Autodesk Inventor part; units mm, degrees
ref_plane "YZ Plane" through (0, 0, 0) normal (1, 0, 0) x (0, 1, 0)
ref_plane "XZ Plane" through (0, 0, 0) normal (0, 1, 0) x (-1, 0, 0)
ref_plane "XY Plane" through (0, 0, 0) normal (0, 0, 1) x (1, 0, 0)
sketch "Sketch1" plane through (0, 0, 0) normal (0, 0, 1) x (1, 0, 0)
  line L0 (-21.5, 19) -> (21.5, 19)
  line L1 (21.5, 19) -> (21.5, -19)
  line L2 (21.5, -19) -> (-21.5, -19)
  line L3 (-21.5, -19) -> (-21.5, 19)
  line L4 (0, 0) -> (0, 19) construction
  line L5 (0, 0) -> (0, -19) construction
  line L6 (0, 0) -> (21.5, 0) construction
  line L7 (0, 0) -> (-21.5, 0) construction
  dimension "d0" = 43
  dimension "d1" = 38
extrude "Extrusion1" add sketch "Sketch1" along normal blind 4.5
sketch "Sketch2" plane through (0, 0, 4.5) normal (0, 0, 1) x (1, 0, 0)
  line L0 (21.5, 19) -> (21.5, -19)
  line L1 (-21.5, 19) -> (21.5, 19)
  line L2 (-21.5, -19) -> (-21.5, 19)
  line L3 (21.5, -19) -> (-21.5, -19)
  line L4 (19.7, 17.2) -> (19.7, -17.2)
  line L5 (19.7, -17.2) -> (-19.7, -17.2)
  line L6 (-19.7, -17.2) -> (-19.7, 17.2)
  line L7 (-19.7, 17.2) -> (19.7, 17.2)
  dimension "d4" = 1.8
extrude "Extrusion2" cut sketch "Sketch2" against normal blind 2.25 contours L4 L5 L6 L7
sketch "Sketch3" plane through (0, 0, 0) normal (0, 0, -1) x (-1, 0, 0)
  line L0 (21.5, 19) -> (-21.5, 19)
  line L1 (-21.5, 19) -> (-21.5, -19)
  line L2 (-21.5, 17) -> (-23.5, 17)
  line L3 (-23.5, 17) -> (-23.5, 12.725)
  line L4 (-23.5, 12.725) -> (-34.5, 12.725)
  line L5 (-34.5, 12.725) -> (-34.5, 2.425)
  line L6 (-34.5, 2.425) -> (-23.5, 2.425)
  line L7 (-23.5, 2.425) -> (-23.5, -1.85)
  line L8 (-23.5, -1.85) -> (-21.5, -1.85)
  dimension "d7" = 2
  dimension "d8" = 2
  dimension "d9" = 18.85
  dimension "d10" = 10.3
  dimension "d11" = 13
extrude "Extrusion3" add sketch "Sketch3" against normal blind 2
fillet "Fillet1" radius 5.15 2 edges at (34.5, 2.425, 1) (34.5, 12.725, 1)
fillet "Fillet1" radius 2 2 edges at (23.5, 2.425, 1) (23.5, 12.725, 1)
sketch "Sketch4" plane through (0, 0, 2) normal (0, 0, 1) x (1, 0, 0)
  arc A0 (29.35, 2.425) -> (29.35, 12.725) centre (29.35, 7.575) ccw
hole "Hole1" at (29.35, 7.575, 2) direction (0, 0, -1) diameter 5 end through all
sketch "Sketch5" plane through (0, 0, 2) normal (0, 0, 1) x (1, 0, 0)
  line L0 (21.5, -1.85) -> (21.5, 17)
  line L1 (23.5, -1.85) -> (21.5, -1.85)
  line L2 (21.5, -1.85) -> (21.5, -0.5)
  line L3 (21.5, -0.5) -> (23.5, -0.5)
  line L4 (23.5, -0.5) -> (23.5, -1.85)
  line L5 (23.5, 17) -> (21.5, 17)
  line L6 (21.5, 17) -> (21.5, 15.65)
  line L7 (21.5, 15.65) -> (23.5, 15.65)
  line L8 (23.5, 15.65) -> (23.5, 17)
  dimension "d23" = 1.35
extrude "Extrusion4" add sketch "Sketch5" along normal blind 5.15
mirror "Mirror1" about plane through (0, 0, 0) normal (1, 0, 0) of "Extrusion4", "Hole1", "Extrusion3", "Fillet1"
sketch "Sketch6" plane through (0, 0, 2.25) normal (0, 0, 1) x (1, 0, 0)
  circle A0 centre (0, 7.575) radius 2.5
  line L0 (-21.5, 19) -> (21.5, 19)
  circle A1 centre (-29.35, 7.575) radius 2.5
  point P0 (0, 0)
  dimension "d26" = 5
extrude "Extrusion5" add sketch "Sketch6" along normal up to surface (2.25 mm away) contours A0
sketch "Sketch7" plane through (0, 0, 2.25) normal (0, 0, 1) x (1, 0, 0)
  circle A0 centre (-15.9, -11.65) radius 2.5
  circle A1 centre (15.4, -6) radius 2.5
  line L0 (-21.5, -19) -> (-21.5, -1.85)
  line L1 (21.5, -19) -> (-21.5, -19)
  line L2 (21.5, -1.85) -> (21.5, -19)
  dimension "d30" = 5
  dimension "d31" = 5.6
  dimension "d32" = 7.35
  dimension "d33" = 6.1
  dimension "d34" = 13
extrude "Extrusion6" add sketch "Sketch7" along normal up to surface (2.25 mm away)
sketch "Sketch8" plane through (-15.9, -11.65, 4.5) normal (0, 0, 1) x (1, 0, 0)
  circle A0 centre (0, 0) radius 2.5
  circle A1 centre (0, 0) radius 1.5
  circle A2 centre (31.3, 5.65) radius 2.5
  circle A3 centre (31.3, 5.65) radius 1.5
  dimension "d37" = 3
extrude "Extrusion7" add sketch "Sketch8" along normal blind 8 contours A1 | A3
properties part number "Spike Bottom Cover" material "ABS Plastic"
CAD build for the part. Positions are in the model's coordinates, mm. A direction names the side the tool comes from. Give positions to 0.01 mm unless a question says otherwise; leave off trailing zeros. Order: outer loops, then holes, each group sorted by start corner. A loop starts at its lowest first (then second) coordinate and runs counter-clockwise, first axis right, second up.
(1) Mould opens along Y. For faces 1 (the flat face through (0, -19, 2)), 2 (the flat face through (22, 16, 7.15)), 3 (the flat face through (-23, -0.5, 5)) say: released by +Y, released by -Y, zero draft, split by the parting line, or undercut.
(2) Flat gauge pins, fed straight in: pin 1 (1.1 mm diameter, centred on y = 0, z = 5, fed in from -X); pin 2 (5 mm diameter, centred on y = -10, z = 2.5, fed in from -X); pin 3 (1.5 mm diameter, centred on y = -7, z = 7, fed in from -X). Where does each tip first touch, or does it go through?
(3) Tool access for faces 4 (the flat face through (-14, -12, 4.5)), 5 (the flat face through (21.5, 8, 3)), 6 (the flat face through (21.5, 16, 6)), 7 (the flat face through (23.5, -1, 3)), 8 (the flat face through (-23.5, 16, 3)): list every direction of +Z, -Z, +X, -X, +Y, -Y with a clear straight run to the whole face (end or side of a thin tool).
(4) Saw through at B-B, the plane x = 30.5. Give the cut face in (y, z), then the cut area to 3 significant figures.
(5) Saw through at A-A, the plane z = 3. Give the cut face in (x, y) (3 decimals), then the cut area to 3 significant figures.
(6) Drill centre lines: L1, parallel to Y at x = -29.35, z = 0.55 (3 decimals); L2, parallel to X at y = 6.5, z = 1.25; L3, parallel to Y at x = -5, z = 4. Where is each one in solid material? Low to high.
(7) Saw through at D-D, the plane x = -6.5. Give the cut face in (y, z), then the cut area to 3 significant figures.
(8) Saw through at C-C, the plane y = -15. Give the cut face in (x, z).
Results found:
1. face 1: released by -Y
1. face 2: zero draft
1. face 3: undercut
2. pin 1: stops at x = -23.5
2. pin 2: stops at x = -21.5
2. pin 3: stops at x = 13.92
3. face 4: +Z
3. face 5: +Z, +X
3. face 6: +Z, +Y, -Y
3. face 7: +Z, -Z, +X, -Y
3. face 8: +Z, -Z, -X, +Y
4. outline: (2.56, 0) - (5.36, 0) - (5.36, 2) - (2.56, 2) - close; (9.79, 0) - (12.59, 0) - (12.59, 2) - (9.79, 2) - close
4. area: 11.2 mm2
5. outline: (-23.5, -1.85) - (-21.5, -1.85) - (-21.5, -19) - (21.5, -19) - (21.5, -1.85) - (23.5, -1.85) - (23.5, -0.5) - (21.5, -0.5) - (21.5, 15.65) - (23.5, 15.65) - (23.5, 17) - (21.5, 17) - (21.5, 19) - (-21.5, 19) - (-21.5, 17) - (-23.5, 17) - (-23.5, 15.65) - (-21.5, 15.65) - (-21.5, -0.5) - (-23.5, -0.5) - close; circle Ø5 at (-15.9, -11.65); circle Ø5 at (0, 7.575); circle Ø5 at (15.4, -6); hole (-19.7, -17.2) - (19.7, -17.2) - (19.7, 17.2) - (-19.7, 17.2) - close
5. area: 348 mm2
6. L1: y = 2.425 to 5.075, 10.075 to 12.725
6. L2: x = -34.39 to -31.61, -27.09 to 27.09, 31.61 to 34.39
6. L3: y = -19 to -17.2, 17.2 to 19
7. outline: (-19, 0) - (19, 0) - (19, 4.5) - (17.2, 4.5) - (17.2, 2.25) - (-17.2, 2.25) - (-17.2, 4.5) - (-19, 4.5) - close
7. area: 93.6 mm2
8. outline: (-21.5, 0) - (21.5, 0) - (21.5, 4.5) - (19.7, 4.5) - (19.7, 2.25) - (-19.7, 2.25) - (-19.7, 4.5) - (-21.5, 4.5) - close
